Geometry check sheet. Reference: the model listing, model coordinates, mm. Face numbers are marked on the shaded views. A direction names the side the tool comes from. Give positions to 0.01 mm unless a question says otherwise; leave off trailing zeros. Write each loop counter-clockwise with the first axis right and the second up, starting at its lowest first coordinate (ties: lowest second). Pieces come first, ordered by that corner, then holes. Notation, with made-up numbers: (49.25, -2.5) - (101.25, -2.5) arc R12 cw to (101.25, 15.5) - close; hole circle Ø9 at (-34, -18.5). An arc over 180 degrees is marked (long way). Use a Markdown table: item, result.
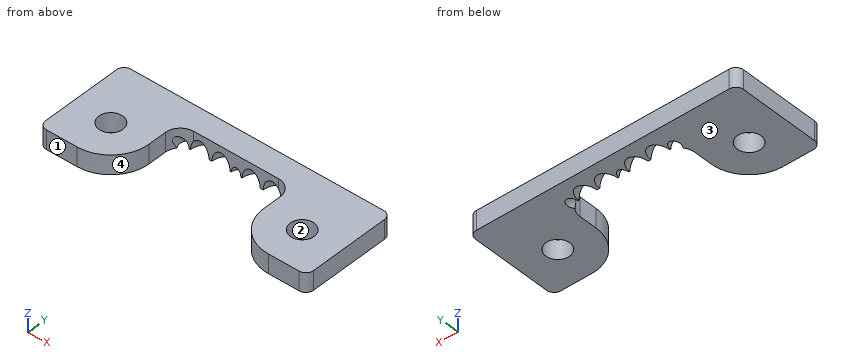
```python
from build123d import *

# Parameters (mm, degrees)
SKETCH2_R                = 3.96875
BOSS_EXTRUDE1_DEPTH      = 6.35
CUT_EXTRUDE1_START       = -1.875700318
CUT_EXTRUDE1_OUTLINE_R   = 3
CUT_EXTRUDE1_OUTLINE_R_2 = 1.59
CUT_EXTRUDE1_DEPTH       = 7.374548908


# Read off the part's stored shape, not the designer's step: Cut-Extrude1
with BuildPart() as part:
    # Sketch2 → Boss-Extrude1 (new body)
    with BuildSketch(Plane.XY):
        with BuildLine():
            Line((2.5, 38.1), (86.4, 38.1))
            ThreePointArc((86.4, 38.1), (88.167766953, 37.367766953), (88.9, 35.6))
            Line((88.9, 35.6), (88.9, 8.85))
            ThreePointArc((88.9, 8.85), (88.167766953, 7.082233047), (86.4, 6.35))
            Line((86.4, 6.35), (76.2, 6.35))
            ThreePointArc((76.2, 6.35), (67.219743879, 10.069743879), (63.5, 19.05))
            Line((63.5, 19.05), (63.5, 25.16))
            ThreePointArc((63.5, 25.16), (62.035533906, 28.695533906), (58.5, 30.16))
            Line((58.5, 30.16), (30.4, 30.16))
            ThreePointArc((30.4, 30.16), (26.864466094, 28.695533906), (25.4, 25.16))
            Line((25.4, 25.16), (25.4, 19.05))
            ThreePointArc((25.4, 19.05), (21.680256121, 10.069743879), (12.7, 6.35))
            Line((12.7, 6.35), (2.5, 6.35))
            ThreePointArc((2.5, 6.35), (0.732233047, 7.082233047), (0, 8.85))
            Line((0, 8.85), (0, 35.6))
            ThreePointArc((0, 35.6), (0.732233047, 37.367766953), (2.5, 38.1))
        make_face()
        with Locations((12.7, 19.05)):
            Circle(SKETCH2_R, mode=Mode.SUBTRACT)
        with Locations((76.2, 19.05)):
            Circle(SKETCH2_R, mode=Mode.SUBTRACT)
    extrude(amount=BOSS_EXTRUDE1_DEPTH)

    # Cut-Extrude1 outline → Cut-Extrude1 (cut)
    with BuildSketch(Plane(origin=(0, 15.875, -15.875), x_dir=(1, 0, 0), z_dir=(0, -0.7071067811865475, 0.7071067811865477)).offset(CUT_EXTRUDE1_START)):
        with Locations((56.45, 21.326340521)):
            Circle(CUT_EXTRUDE1_OUTLINE_R)
        with BuildLine():
            ThreePointArc((52.45, 21.326340521), (49.45, 24.326340521), (46.45, 21.326340521))
            Line((46.45, 21.326340521), (52.45, 21.326340521))
        make_face()
        with BuildLine():
            ThreePointArc((46.04, 21.326340521), (44.45, 22.916340521), (42.86, 21.326340521))
            Line((42.86, 21.326340521), (46.04, 21.326340521))
        make_face()
        with BuildLine():
            ThreePointArc((42.45, 21.326340521), (39.45, 24.326340521), (36.45, 21.326340521))
            Line((36.45, 21.326340521), (42.45, 21.326340521))
        make_face()
        with Locations((32.45, 21.326340521)):
            Circle(CUT_EXTRUDE1_OUTLINE_R)
        with Locations((61.45, 21.326340521)):
            Circle(CUT_EXTRUDE1_OUTLINE_R_2)
        with Locations((27.45, 21.326340521)):
            Circle(CUT_EXTRUDE1_OUTLINE_R_2)
    extrude(amount=CUT_EXTRUDE1_DEPTH, mode=Mode.SUBTRACT)


solid = part.part
```
1) Section check B-B on x = 19. Record the boundary of the cut face in (y, z).
Working result:
| item | result |
|---|---|
| outline | (8.02, 0) - (38.1, 0) - (38.1, 6.35) - (8.02, 6.35) - close |
2) Depth check by flat-ended pin: P1, Ø12.5, axis at x = 12.7, y = 19.05, coming from the -Z side; P2, Ø1.9, axis at x = 46, z = 3.5, coming from the -Y side. Enter the tip coordinate at first touch or a pass-through.
Working result:
| item | result |
|---|---|
| P1 | stops at z = 0 |
| P2 | stops at y = 30.16 |
3) Section check A-A on y = 26. Record the boundary of the cut face in (x, z), then the cut area to 3 significant figures.
Working result:
| item | result |
|---|---|
| outline | (0, 0) - (25.47, 0) - (25.47, 6.35) - (0, 6.35) - close; (63.43, 0) - (88.9, 0) - (88.9, 6.35) - (63.43, 6.35) - close |
| area | 323 mm² |
4) Material ranges on L1, parallel to X at y = 25.5, z = 4; L2, parallel to Y at x = 12.7, z = 4.25; L3, parallel to X at y = 16, z = 4.25, recorded low to high. Write a range as from..to.
Working result:
| item | result |
|---|---|
| L1 | x = 0..25.41, 63.49..88.9 |
| L2 | y = 6.35..15.08, 23.02..38.1 |
| L3 | x = 0..10.16, 15.24..25.03, 63.87..73.66, 78.74..88.9 |
5) Section check D-D on x = 38. Record the boundary of the cut face in (y, z), then the cut area to 3 significant figures.
Working result:
| item | result |
|---|---|
| outline | (30.16, 3.71) - (33.87, 0) - (38.1, 0) - (38.1, 6.35) - (30.16, 6.35) - close |
| area | 43.5 mm² |
6) Section check C-C on z = 1.25. Count the separate pieces of the cut face and the enclosed holes in it, then the cut area to 3 significant figures.
Working result:
| item | result |
|---|---|
| separate pieces | 1 |
| enclosed holes | 2 |
| area | 1,690 mm² |
7) Mould release check, pull along X, two halves, no side actions. Record for the marked faces 1 and 2: pulls with the +X half, pulls with the -X half, needs draft (parallel to the pull), parting line crosses it, or undercut.
Working result:
| item | result |
|---|---|
| face 1 | needs draft |
| face 2 | undercut |
8) Set-up check for the marked faces 3 and 4: record each of +Z, -Z, +X, -X, +Y, -Y from which the full face is reachable in a straight line by a thin tool's end or side.
Working result:
| item | result |
|---|---|
| face 3 | -Z, +X, -X, +Y, -Y |
| face 4 | +Z, -Z, -Y |
